from build123d import *

# Parameters (mm, degrees)
F4_DEPTH      = 45.391737605
F4_DEPTH_BACK = 45.391737605
F6_DEPTH      = 45.391737605
F7_DEPTH      = 45.391737605


with BuildPart() as f2:
    # F0 (on Front) → F2 (revolve)
    with BuildSketch(Plane.XZ):
        with BuildLine():
            Line((0, 45.390737605), (0, -45.390737605))
            ThreePointArc((0, -45.390737605), (45.390737605, 0), (0, 45.390737605))
        make_face()
    revolve(axis=Axis((0, 0, -0.1771636307), (0, 0, -1)))

    # F3 (on Front) → F4 (cut, two sides)
    with BuildSketch(Plane.XZ) as f4_sk:
        Polygon((0, -20.2791038901), (-40.3937026858, -20.2791038901), (-40.3937026858, -45.9680799395), (0, -45.9680799395), (40.3937026858, -45.9680799395), (40.3937026858, -20.2791038901), align=None)
    extrude(amount=-F4_DEPTH, mode=Mode.SUBTRACT)
    extrude(f4_sk.sketch, amount=F4_DEPTH_BACK, mode=Mode.SUBTRACT)

    # F5 (on Front) → F6 (cut, through all)
    with BuildSketch(Plane.XZ):
        Polygon((9.3581555411, 46.5339459479), (4.3016839772, 46.5339459479), (47.9137524962, 2.0791364368), (50.4419840872, 46.5339459479), align=None)
    extrude(amount=F6_DEPTH, mode=Mode.SUBTRACT)

    # F5 (on Front) → F7 (cut, through all)
    with BuildSketch(Plane.XZ):
        Polygon((9.3581555411, 46.5339459479), (4.3016839772, 46.5339459479), (47.9137524962, 2.0791364368), (50.4419840872, 46.5339459479), align=None)
    extrude(amount=-F7_DEPTH, mode=Mode.SUBTRACT)


solid = f2.part
Geometry: final body of the model. Coordinates: model frame, mm. A direction names the side the tool comes from. Coordinates: 2 decimals unless noted, no trailing zeros. Loops run counter-clockwise (first coordinate to the right, second up) from the corner with the lowest first, then second, coordinate; pieces in that order, holes last. Notation, with made-up numbers: (13.5, 69.25) - (23.5, 69.25) arc R24 cw to (23.5, 84.25) - close; hole circle Ø6 at (69.25, -23). An arc over 180 degrees is marked (long way). One line per question, with ' | ' between items. Start each with the question number.
(1) First-contact query: pin 1 (1 mm diameter, centred on x = -9, z = -13, fed in from -Y); pin 2 (5 mm diameter, centred on y = -7.5, z = 22, fed in from +X); pin 3 (4 mm diameter, centred on y = -7.5, z = -13, fed in from +X). Flat tips, straight axial feed; report the tip coordinate or a pass-through.
(2) Cut plane C-C on z = -17. Output: boundary loops of the cut face in (x, y), and give its area (3 significant figures).
(3) Reachability of faces 1 (the flat face through (1, -1, -20.279)), 2 (the flat face through (25.18, 0.39, 25.25)) from +Z, -Z, +X, -X, +Y, -Y: full face, straight path, thin tool, end or side. Return the list, or none.
(4) Cut plane D-D on z = 2. Output: boundary loops of the cut face in (x, y).
(5) Cut plane B-B on y = 30.5. Output: boundary loops of the cut face in (x, z), and give its area (3 significant figures).
(6) Ray query, L1, parallel to Z at x = -34.5, y = -9; L2, parallel to Z at x = 25.5, y = -22.5; L3, parallel to X at y = -35, z = 10. Return the intervals inside material, ascending. Write a range as from..to.
(7) Cut plane A-A on x = -2.5. Output: boundary loops of the cut face in (y, z).
Here are the results:
1) pin 1: y = -42.73 | pin 2: x = 30.82 | pin 3: x = 43.49
2) outline: circle Ø84.17 at (0, 0) | area: 5,560 mm²
3) face 1: -Z, +Y, -Y | face 2: +Z, +X, +Y, -Y
4) outline: circle Ø90.69 at (0, 0)
5) outline: (-26.81, -20.28) - (26.81, -20.28) arc R33.62 ccw (long way) to start | area: 3,050 mm²
6) L1: -20.28..28.09 | L2: -20.28..24.93 | L3: -27.12..27.12
7) outline: (-40.53, -20.28) - (40.53, -20.28) arc R45.32 ccw (long way) to start
